The listing builds one solid part. Answer for the finished solid, in the listing's coordinates (mm). Face numbers are marked on the shaded views. A direction names the side the tool comes from. Give positions to 0.01 mm unless a question says otherwise; leave off trailing zeros. Loops run counter-clockwise (first coordinate to the right, second up) from the corner with the lowest first, then second, coordinate; pieces in that order, holes last. Notation, with made-up numbers: (87, -30.5) -> (122, -30.5) arc R15 ccw to (122, -9.5) -> close; hole circle Ø9 at (-13, -24.75). An arc over 180 degrees is marked (long way). One line per question, with ' | ' between items. Start each with the question number.
from build123d import *

# Parameters (mm, degrees)
F1_DEPTH = 63.5
F2_W     = 38.1
F2_H     = 50.8
F3_DEPTH = 25.4


with BuildPart() as f1:
    # F0 (on Front) → F1 (new body)
    with BuildSketch(Plane.XZ):
        Polygon((-86.982761, -25.590784), (-10.782761, -25.590784), (-10.782761, -0.190784), (-61.582761, -0.190784), (-61.582761, 50.609216), (-86.982761, 50.609216), (-125.082761, 50.609216), (-125.082761, 22.604095), (-86.982761, 22.604095), align=None)
    extrude(amount=F1_DEPTH)

    # F2 (on face) → F3 (join)
    with BuildSketch(Plane.XZ.offset(63.5)):
        with Locations((-42.532761, 25.209216)):
            Rectangle(F2_W, F2_H)
    extrude(amount=-F3_DEPTH)


solid = f1.part
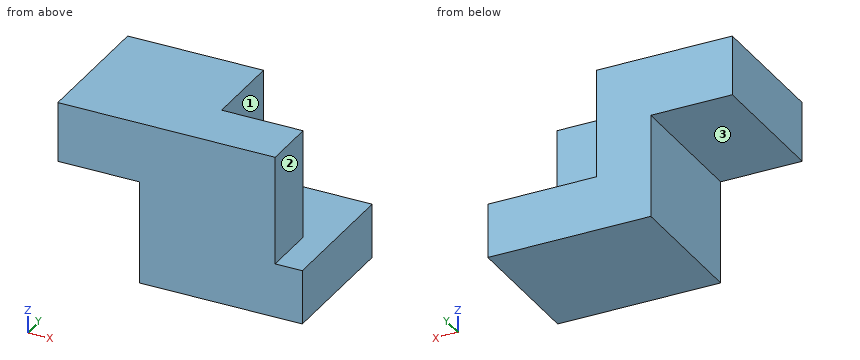
1. The part is cut by section C-C (x = -47.5). Write down the section's boundary in (y, z), plus the area to 3 significant figures.
2. The part is cut by section A-A (y = -7). Write down the section's boundary in (x, z).
3. The part is cut by section D-D (y = -58.5). Write down the section's boundary in (x, z), plus the area to 3 significant figures.
4. Each of these flat-tipped pins is pushed along its axis until it touches: pin 1 Ø1.5 at (x, y) = (-44.5, -35.5) entering from +Z; pin 2 Ø20.5 at (y, z) = (-50, 35.5) entering from +X; pin 3 Ø4 at (y, z) = (-15, 20) entering from +X; pin 4 Ø12 at (x, z) = (-90.5, -11) entering from -Y. Where does it stop, or does it pass through?
5. The part is cut by section B-B (z = 10.5). Write down the section's boundary in (x, y).
6. Straight lines are drawn through the part: L1, parallel to X at y = -57, z = -5; L2, parallel to X at y = -15.5, z = 41.5; L3, parallel to Z at x = -30.5, y = -7. For each, find the intervals that lie inside material, in ascending order.
7. For the marked faces 1, 2 and 3, determine the directions among +Z, -Z, +X, -X, +Y, -Y from which every point of the face is accessible in a straight line to the end or side of a thin tool.
Check sheet entries:
1) outline: (-63.5, -25.59) -> (0, -25.59) -> (0, -0.19) -> (-38.1, -0.19) -> (-38.1, 50.61) -> (-63.5, 50.61) -> close | area: 2,900 mm^2
2) outline: (-125.08, 22.6) -> (-86.98, 22.6) -> (-86.98, -25.59) -> (-10.78, -25.59) -> (-10.78, -0.19) -> (-61.58, -0.19) -> (-61.58, 50.61) -> (-125.08, 50.61) -> close
3) outline: (-125.08, 22.6) -> (-86.98, 22.6) -> (-86.98, -25.59) -> (-10.78, -25.59) -> (-10.78, -0.19) -> (-23.48, -0.19) -> (-23.48, 50.61) -> (-125.08, 50.61) -> close | area: 6,230 mm^2
4) pin 1: stops at z = -0.19 | pin 2: stops at x = -23.48 | pin 3: stops at x = -61.58 | pin 4: stops at y = -63.5
5) outline: (-86.98, -63.5) -> (-23.48, -63.5) -> (-23.48, -38.1) -> (-61.58, -38.1) -> (-61.58, 0) -> (-86.98, 0) -> close
6) L1: x = -86.98 to -10.78 | L2: x = -125.08 to -61.58 | L3: z = -25.59 to -0.19
7) face 1: +Z, +X, +Y | face 2: +Z, +X, +Y, -Y | face 3: -Z, -X, +Y, -Y
